Design review of the part built by this model. Coordinates are the model's own, in mm. A direction names the side the tool comes from. Give positions to 0.01 mm unless a question says otherwise; leave off trailing zeros. Order: outer loops, then holes, each group sorted by start corner. A loop starts at its lowest first (then second) coordinate and runs counter-clockwise, first axis right, second up. Notation, with made-up numbers: M 27,67.5 L 48,67.5 A25 cw 48,93.5 Z; hole C 36.25,-0.75 d4. An arc over 180 degrees is marked long. Answer as a JSON object with one key per item and string values.
from build123d import *

# Parameters (mm, degrees)
SKETCH1_R           = 3.4
SKETCH1_R_2         = 2.4
BOSS_EXTRUDE1_DEPTH = 3.5
SKETCH2_R           = 3.4
SKETCH2_R_2         = 1.5
BOSS_EXTRUDE2_DEPTH = 8.5
CUT_EXTRUDE1_START  = -6.5
SKETCH3_R           = 2.5
SKETCH3_R_2         = 1.5
CUT_EXTRUDE1_DEPTH  = 6.5
SKETCH4_R           = 1.5
SKETCH4_R_2         = 2.5
BOSS_EXTRUDE3_DEPTH = 2.5
CHAMFER_1_SIZE      = 0.1
CHAMFER_1_SIZE2     = 8


with BuildPart() as part:
    # Sketch1 → Boss-Extrude1 (new body)
    with BuildSketch(Plane.XY):
        Circle(SKETCH1_R)
        Circle(SKETCH1_R_2, mode=Mode.SUBTRACT)
    extrude(amount=BOSS_EXTRUDE1_DEPTH)

    # Sketch2 → Boss-Extrude2 (add)
    with BuildSketch(Plane.XY.offset(3.5)):
        Circle(SKETCH2_R)
        Circle(SKETCH2_R_2, mode=Mode.SUBTRACT)
    extrude(amount=BOSS_EXTRUDE2_DEPTH)

    # Sketch3 → Cut-Extrude1 (cut)
    with BuildSketch(Plane.XY.offset(12).offset(CUT_EXTRUDE1_START)):
        Circle(SKETCH3_R)
        Circle(SKETCH3_R_2, mode=Mode.SUBTRACT)
    extrude(amount=CUT_EXTRUDE1_DEPTH, mode=Mode.SUBTRACT)

    # Sketch4 → Boss-Extrude3 (add)
    with BuildSketch(Plane.XY.offset(12)):
        with BuildLine():
            Line((-2.794955456, 10.168), (-3.393874482, 0.204))
            ThreePointArc((-3.393874482, 0.204), (0, -3.4), (3.393874482, 0.204))
            Line((3.393874482, 0.204), (2.794955456, 10.168))
            ThreePointArc((2.794955456, 10.168), (0, 12.8), (-2.794955456, 10.168))
        make_face()
        with Locations((0, 10)):
            Circle(SKETCH4_R, mode=Mode.SUBTRACT)
        Circle(SKETCH4_R_2, mode=Mode.SUBTRACT)
    extrude(amount=BOSS_EXTRUDE3_DEPTH)

    # 倒角1
    chamfer_1_edges = [part.edges().sort_by_distance(p)[0] for p in [
        (-3.4, 0, 0),
    ]]
    chamfer_1_side = [part.faces().sort_by_distance(p)[0] for p in [
        (-3.303833478, 0, 0),
    ]]
    chamfer(chamfer_1_edges, length=CHAMFER_1_SIZE, length2=CHAMFER_1_SIZE2, reference=chamfer_1_side[0])


solid = part.part
(1) Tool access review of faces 4 (the flat face through (0, -2, 5.5)), 5 (the conical face through (-0.44, 3.32, 4.06)), 6 (the cylindrical face through (-0.325, 8.536, 13.232)): name each direction out of +Z, -Z, +X, -X, +Y, -Y from which nothing blocks a thin tool from reaching the whole face with its end or side.
Checked values:
{"face 4": "+Z", "face 5": "-Z", "face 6": "+Z, -Z"}
(2) We need section B-B (x = 0). Count the separate pieces of the cut face and the enclosed holes in it, plus the area to 3 significant figures.
Checked values:
{"separate pieces": "3", "enclosed holes": "0", "area": "46.0 mm^2"}
(3) We need section C-C (y = 5.25). Write out the cut boundary in (x, z), plus the area to 3 significant figures.
Checked values:
{"outline": "M -3.09,12 L 3.09,12 L 3.09,14.5 L -3.09,14.5 Z", "area": "15.5 mm^2"}
(4) Draft analysis for pull direction Y (two halves, no side actions). For faces 1 (the flat face through (0, 5, 14.5)), 2 (the flat face through (-3.09, 5.26, 13.23)), 3 (the cylindrical face through (1.29, 2.024, 1.726)), state which applies: +Y half, -Y half, draft (parallel to the pull), parting line (faces both ways), or undercut.
Checked values:
{"face 1": "draft", "face 2": "+Y half", "face 3": "undercut"}
(5) To check wall thickness, follow L1, parallel to Z at x = -1.25, y = 5; L2, parallel to Y at x = -1.75, z = 9.5; L3, parallel to Y at x = -1.5, z = 10. State the ranges of each line that lie inside material, in increasing order. Write a range as from..to.
Checked values:
{"L1": "z = 12..14.5", "L2": "y = -2.92..-1.79, 1.79..2.92", "L3": "y = -3.05..-2, 2..3.05"}
(6) We need section A-A (z = 10.75). Write out the cut boundary in (x, y).
Checked values:
{"outline": "C 0,0 d6.8; hole C 0,0 d5"}
(7) We need section D-D (z = 4). Write out the cut boundary in (x, y).
Checked values:
{"outline": "C 0,0 d6.7; hole C 0,0 d3"}
(8) Insertion check: pin 1 (1 mm diameter, centred on x = -0.5, y = 0, fed in from -Z); pin 2 (1.5 mm diameter, centred on x = 1, z = 2, fed in from +Y); pin 3 (4 mm diameter, centred on x = 0, y = 10, fed in from -Z); pin 4 (2 mm diameter, centred on y = 2, z = 6.5, fed in from +X). Each pin has a flat end and moves straight along its axis. Give the tip position at first contact, or say it passes through.
Checked values:
{"pin 1": "passes through", "pin 2": "stops at y = 3.32", "pin 3": "stops at z = 12", "pin 4": "stops at x = 3.23"}
